Verification items for the finished model (mm, model axes). Coordinates: 2 decimals unless noted, no trailing zeros. Write each loop counter-clockwise with the first axis right and the second up, starting at its lowest first coordinate (ties: lowest second). Pieces come first, ordered by that corner, then holes. Notation, with made-up numbers: (53, 1) - (62, 1) arc R31 ccw to (62, 39) - close; hole circle Ø8 at (32.25, 88). An arc over 180 degrees is marked (long way). Use one line per item in the form item = value. Start each with the question number.
(1) Sectioned sample at D-D (x = -82.5). Record the cut outline in (y, z), and give its area (3 significant figures).
(2) Gauge pin test, flat ends, axial feed: pin 1 Ø2.5 at (x, y) = (-95.95, 73.59) entering from +Z; pin 2 Ø1 at (x, z) = (-44, 1.5) entering from -Y. Record the tip position at first contact, or that the pin passes through.
(3) Sectioned sample at A-A (x = -15). Record the cut outline in (y, z).
(4) Material ranges on line 1 (Y direction, x = -91, z = 0.4); line 2 (Y direction, x = -15, z = 2.75); line 3 (X direction, y = 15.5, z = 0.65), recorded low to high. Write a range as [from, to].
(5) Sectioned sample at C-C (y = 18). Record the cut outline in (x, z), and give its area (3 significant figures).
(6) Sectioned sample at B-B (z = 1.7). Record the cut outline in (x, y), and give its area (3 significant figures).
(7) Mould release check, pull along Y, two halves, no side actions. Record for faces 1 (the flat face through (-57.766, 31.689, 1.972)), 2 (the flat face through (-48, 38, 0)), 3 (the cylindrical face through (-94.743, 75.485, 1.972)): released by +Y, released by -Y, zero draft, split by the parting line, or undercut.
from build123d import *

# Parameters (mm, degrees)
SKETCH_R   = 1.1
SKETCH_R_2 = 2.25
SKETCH_R_3 = 1.55
PAD_DEPTH  = 4


with BuildPart() as part:
    # Sketch → Pad (new body)
    with BuildSketch(Plane.XY):
        with BuildLine():
            Line((-20, 0), (0, 0))
            Line((0, 0), (0, 15))
            Line((0, 15), (-86.897903, 75.846567))
            Line((-86.897903, 75.846567), (-93.096869, 79.602543))
            ThreePointArc((-93.096869, 79.602543), (-95.613656, 80.893196), (-96.904309, 78.37641))
            Line((-96.804881, 77.239939), (-96.904309, 78.37641))
            ThreePointArc((-96.804881, 77.239939), (-98.825686, 75.998429), (-99.697425, 73.792739))
            Line((-99.697425, 73.792739), (-100.833896, 73.69331))
            ThreePointArc((-100.833896, 73.69331), (-103.088327, 71.985229), (-101.380247, 69.730798))
            Line((-96.604444, 64.278761), (-101.380247, 69.730798))
            Line((-20, 0), (-96.604444, 64.278761))
        make_face()
        with Locations((-91.751398, 70.062397)):
            Circle(SKETCH_R, mode=Mode.SUBTRACT)
        with Locations((-95.000589, 78.989476)):
            Circle(SKETCH_R, mode=Mode.SUBTRACT)
        with Locations((-101.107072, 71.712054)):
            Circle(SKETCH_R, mode=Mode.SUBTRACT)
        with Locations((-95.95302, 73.587976)):
            Circle(SKETCH_R_2, mode=Mode.SUBTRACT)
        with Locations((-15, 15)):
            Circle(SKETCH_R_3, mode=Mode.SUBTRACT)
    extrude(amount=PAD_DEPTH)


solid = part.part
Answers below:
q1.outline = (52.44, 0) - (72.77, 0) - (72.77, 4) - (52.44, 4) - close
q1.area = 81.3 mm2
q2.pin_1 = through
q2.pin_2 = 19.72
q3.outline = (0, 0) - (13.45, 0) - (13.45, 4) - (0, 4) - close; (16.55, 0) - (25.5, 0) - (25.5, 4) - (16.55, 4) - close
q4.line_1 = [59.58, 69.26], [70.87, 78.33]
q4.line_2 = [0, 13.45], [16.55, 25.5]
q4.line_3 = [-38.47, -16.47], [-13.53, -0.71]
q5.outline = (-41.45, 0) - (-4.28, 0) - (-4.28, 4) - (-41.45, 4) - close
q5.area = 149 mm2
q6.outline = (-101.38, 69.73) - (-96.6, 64.28) - (-20, 0) - (0, 0) - (0, 15) - (-86.9, 75.85) - (-93.1, 79.6) arc R2 ccw to (-96.9, 78.38) - (-96.8, 77.24) arc R3.75 ccw to (-99.7, 73.79) - (-100.83, 73.69) arc R2 ccw to start; hole circle Ø2.2 at (-101.11, 71.71); hole circle Ø4.5 at (-95.95, 73.59); hole circle Ø2.2 at (-95, 78.99); hole circle Ø2.2 at (-91.75, 70.06); hole circle Ø3.1 at (-15, 15)
q6.area = 2,260 mm2
q7.face_1 = released by -Y
q7.face_2 = zero draft
q7.face_3 = undercut
